from build123d import *

# Parameters (mm, degrees)
F0_R     = 36.5696932785
F0_R_2   = 20.2309994717
F1_DEPTH = 25
F2_R     = 5
F3_R     = 5
F4_R     = 5
F5_R     = 5
F6_DEPTH = 25


with BuildPart() as f1:
    # F0 (on Front) → F1 (new body)
    with BuildSketch(Plane.XZ):
        Circle(F0_R)
        Circle(F0_R_2, mode=Mode.SUBTRACT)
    extrude(amount=F1_DEPTH)

    # F2
    f2_edges = [f1.edges().sort_by_distance(p)[0] for p in [
        (-20.230999, -25, 0),
    ]]
    fillet(f2_edges, radius=F2_R)

    # F3
    f3_edges = [f1.edges().sort_by_distance(p)[0] for p in [
        (-20.230999, 0, 0),
    ]]
    fillet(f3_edges, radius=F3_R)

    # F4
    f4_edges = [f1.edges().sort_by_distance(p)[0] for p in [
        (-36.569693, 0, 0),
    ]]
    fillet(f4_edges, radius=F4_R)

    # F5
    f5_edges = [f1.edges().sort_by_distance(p)[0] for p in [
        (-36.569693, -25, 0),
    ]]
    fillet(f5_edges, radius=F5_R)

    # F6 (add): a face of the model
    f6_faces = [f1.faces().sort_by_distance(p)[0] for p in [
        (-30.6767675107, -25, 0),
    ]]
    extrude(f6_faces, amount=F6_DEPTH)


solid = f1.part
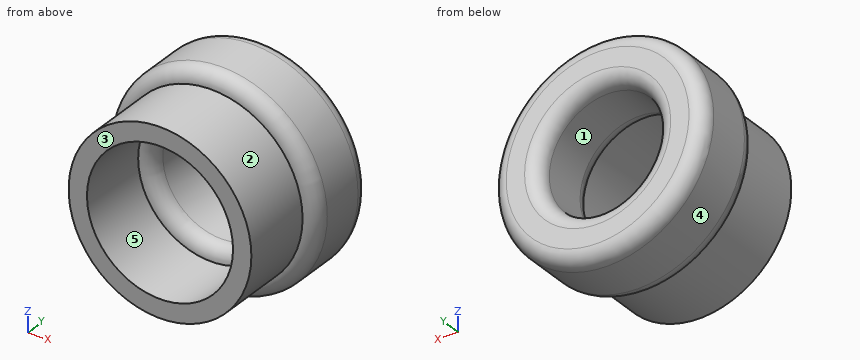
Source: CAD feature listing. Evaluate the final solid. Frame: model axes, mm. Face numbers are marked on the shaded views. A direction names the side the tool comes from. Round coordinates to 2 decimals unless told otherwise and drop trailing zeros. Write each loop counter-clockwise with the first axis right and the second up, starting at its lowest first coordinate (ties: lowest second). Pieces come first, ordered by that corner, then holes. Notation, with made-up numbers: (-34.5, 70) - (-4.5, 70) arc R24 cw to (-4.5, 85) - close; hole circle Ø8 at (16.25, -26). An arc over 180 degrees is marked (long way). Use CSV: the item, a comma, the result in double quotes. Start each with the question number.
(1) Mould query, pull axis X, two halves, no side actions, for the marked faces 1, 2 and 3. Classes: pulls with the +X half, pulls with the -X half, needs draft (parallel to the pull), parting line crosses it, or undercut.
(2) First-contact query: pin 1 Ø2 at (x, z) = (-7, 16.5) entering from +Y; pin 2 Ø4 at (y, z) = (-6, 4) entering from +X; pin 3 Ø3 at (y, z) = (-12, -5) entering from -X; pin 4 Ø6 at (y, z) = (-23.5, -22.5) entering from +X. Flat tips, straight axial feed; report the tip coordinate or a pass-through.
(3) Cut plane D-D, the plane y = -16. Return loops of the section in (x, z).
(4) Cut plane C-C, the plane y = -38.5. Return loops of the section in (x, z).
(5) Cut plane A-A, the plane x = 0. Return loops of the section in (y, z), and give its area (3 significant figures).
(6) Set-up query: the marked faces 4 and 5. Return all of +Z, -Z, +X, -X, +Y, -Y with unobstructed straight access to the full face (end or side cutting, diameter ignored); none if empty.
(7) Material intervals for probe 1 along Z at (x, y) = (0, -31); probe 2 along Z at (x, y) = (0, -9); probe 3 along X at (y, z) = (-30, -15), sorted ascending. Write a range as [from, to].
(8) Cut plane B-B, the plane z = 0. Return loops of the section in (x, y), and give its area (3 significant figures).
Geometry says:
1,face 1,"undercut"
1,face 2,"parting line crosses it"
1,face 3,"needs draft"
2,pin 1,"through"
2,pin 2,"x = 36.51"
2,pin 3,"x = -36.4"
2,pin 4,"x = 30.2"
3,outline,"circle Ø73.14 at (0, 0); hole circle Ø40.46 at (0, 0)"
4,outline,"circle Ø63.14 at (0, 0); hole circle Ø50.46 at (0, 0)"
5,outline,"(-50, -31.57) - (-25, -31.57) arc R5 ccw to (-20, -36.57) - (-5, -36.57) arc R5 ccw to (0, -31.57) - (0, -25.23) arc R5 ccw to (-5, -20.23) - (-20, -20.23) arc R5 ccw to (-25, -25.23) - (-50, -25.23) - close; (-50, 25.23) - (-25, 25.23) arc R5 ccw to (-20, 20.23) - (-5, 20.23) arc R5 ccw to (0, 25.23) - (0, 31.57) arc R5 ccw to (-5, 36.57) - (-20, 36.57) arc R5 ccw to (-25, 31.57) - (-50, 31.57) - close"
5,area,"1,090 mm²"
6,face 4,"+Y, -Y"
6,face 5,"-Y"
7,probe 1,"[-31.57, -25.23], [25.23, 31.57]"
7,probe 2,"[-36.57, -20.23], [20.23, 36.57]"
7,probe 3,"[-27.78, -20.29], [20.29, 27.78]"
8,outline,"(-36.57, -20) arc R5 ccw to (-31.57, -25) - (-31.57, -50) - (-25.23, -50) - (-25.23, -25) arc R5 ccw to (-20.23, -20) - (-20.23, -5) arc R5 ccw to (-25.23, 0) - (-31.57, 0) arc R5 ccw to (-36.57, -5) - close; (20.23, -20) arc R5 ccw to (25.23, -25) - (25.23, -50) - (31.57, -50) - (31.57, -25) arc R5 ccw to (36.57, -20) - (36.57, -5) arc R5 ccw to (31.57, 0) - (25.23, 0) arc R5 ccw to (20.23, -5) - close"
8,area,"1,090 mm²"
